Read the model definition and answer for the solid it produces. Units are mm, in the model's axes. Face numbers are marked on the shaded views. Give positions to 0.01 mm unless a question says otherwise; leave off trailing zeros. Order: outer loops, then holes, each group sorted by start corner. A loop starts at its lowest first (then second) coordinate and runs counter-clockwise, first axis right, second up. Notation, with made-up numbers: (84, 10.25) -> (112, 10.25) arc R9 ccw to (112, 27.25) -> close; hole circle Ø5 at (14.25, 41). An arc over 180 degrees is marked (long way). One line per item, written item: value. Start each with the question number.
from build123d import *

# Parameters (mm, degrees)
CROQUIS1_R              = 49
CROQUIS1_R_2            = 47
SALIENTE_EXTRUIR1_DEPTH = 38
CROQUIS2_R              = 49
CROQUIS2_R_2            = 5
SALIENTE_EXTRUIR3_DEPTH = 2
SALIENTE_EXTRUIR4_START = 15
CROQUIS3_R              = 49
CROQUIS3_R_2            = 45
SALIENTE_EXTRUIR4_DEPTH = 2


with BuildPart() as part:
    # Croquis1 → Saliente-Extruir1 (new body)
    with BuildSketch(Plane.XY):
        Circle(CROQUIS1_R)
        Circle(CROQUIS1_R_2, mode=Mode.SUBTRACT)
    extrude(amount=SALIENTE_EXTRUIR1_DEPTH)

    # Croquis2 → Saliente-Extruir3 (add)
    with BuildSketch(Plane.XY):
        Circle(CROQUIS2_R)
        Circle(CROQUIS2_R_2, mode=Mode.SUBTRACT)
    extrude(amount=SALIENTE_EXTRUIR3_DEPTH)

    # Croquis3 → Saliente-Extruir4 (add)
    with BuildSketch(Plane.XY.offset(SALIENTE_EXTRUIR4_START)):
        Circle(CROQUIS3_R)
        Circle(CROQUIS3_R_2, mode=Mode.SUBTRACT)
    extrude(amount=SALIENTE_EXTRUIR4_DEPTH)


solid = part.part
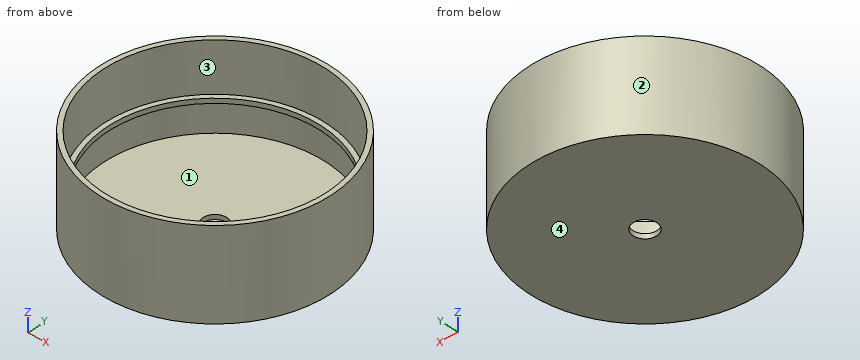
Item 1: Find section C-C on z = 22. Write down the section's boundary in (x, y), then the cut area to 3 significant figures.
Item 2: Find section D-D on y = 26. Write down the section's boundary in (x, z), then the cut area to 3 significant figures.
Item 3: Flat-ended cylindrical pins translate along their axes: pin 1 (5 mm diameter, centred on x = -17.5, y = -34, fed in from -Z); pin 2 (2 mm diameter, centred on x = -17.5, z = 13.5, fed in from +Y); pin 3 (3 mm diameter, centred on y = 32.5, z = 32.5, fed in from -X); pin 4 (9 mm diameter, centred on x = 0, y = 0, fed in from +Z). Find the tip coordinate at first contact, or state that the pin passes through.
Item 4: For a pull along Y with two mould halves and no side action, classify the marked faces 1, 2, 3 and 4 as +Y half, -Y half, draft (parallel to the pull), parting line (faces both ways), or undercut.
Item 5: Find section A-A on y = 0. Write down the section's boundary in (x, z), then the cut area to 3 significant figures.
Item 6: Find the intervals of material crossed by line 1 (Z direction, x = -17, y = 43.5); line 2 (Y direction, x = 0, z = 16.2); line 3 (Y direction, x = 0, z = 7), in increasing order. Write a range as from..to.
Checks:
1. outline: circle Ø98 at (0, 0); hole circle Ø94 at (0, 0)
1. area: 603 mm2
2. outline: (-41.53, 0) -> (41.53, 0) -> (41.53, 38) -> (39.15, 38) -> (39.15, 17) -> (36.73, 17) -> (36.73, 15) -> (39.15, 15) -> (39.15, 2) -> (-39.15, 2) -> (-39.15, 15) -> (-36.73, 15) -> (-36.73, 17) -> (-39.15, 17) -> (-39.15, 38) -> (-41.53, 38) -> close
2. area: 347 mm2
3. pin 1: z = 0
3. pin 2: y = 46.14
3. pin 3: x = -37.95
3. pin 4: through
4. face 1: undercut
4. face 2: parting line
4. face 3: undercut
4. face 4: draft
5. outline: (-49, 0) -> (-5, 0) -> (-5, 2) -> (-47, 2) -> (-47, 15) -> (-45, 15) -> (-45, 17) -> (-47, 17) -> (-47, 38) -> (-49, 38) -> close; (5, 0) -> (49, 0) -> (49, 38) -> (47, 38) -> (47, 17) -> (45, 17) -> (45, 15) -> (47, 15) -> (47, 2) -> (5, 2) -> close
5. area: 328 mm2
6. line 1: 0..2, 15..17
6. line 2: -49..-45, 45..49
6. line 3: -49..-47, 47..49
